Here's how the part is built. I have some questions about the finished solid (model axes, mm). A direction names the side the tool comes from. Round coordinates to 2 decimals unless told otherwise and drop trailing zeros. Loops run counter-clockwise (first coordinate to the right, second up) from the corner with the lowest first, then second, coordinate; pieces in that order, holes last. Notation, with made-up numbers: (2, 58.25) - (32, 58.25) arc R6 ccw to (32, 68.25) - close; hole circle Ø3 at (3.25, 74.25). An arc over 180 degrees is marked (long way). Return JSON: item names as keys, results as strings. Group by question number.
```python
from build123d import *

# Parameters (mm, degrees)
SKETCH1_R           = 1.5
BOSS_EXTRUDE1_DEPTH = 10
SKETCH2_R           = 4
BOSS_EXTRUDE2_DEPTH = 3
SKETCH3_W           = 1.5
SKETCH3_H           = 1
SKETCH3_W_2         = 1
SKETCH3_H_2         = 1.5
CUT_EXTRUDE1_DEPTH  = 2
FILLET1_SIZE        = 2
FILLET1_SIZE_2      = 3.5


with BuildPart() as part:
    # Sketch1 → Boss-Extrude1 (new body)
    with BuildSketch(Plane(origin=(0, 0, 0), x_dir=(1, 0, 0), z_dir=(0, 1, 0))):
        with Locations(Location((0, 0, 0), (0, 0, 270))):
            Circle(SKETCH1_R)
    extrude(amount=BOSS_EXTRUDE1_DEPTH)

    # Sketch2 → Boss-Extrude2 (add)
    with BuildSketch(Plane(origin=(0, 10, 0), x_dir=(1, 0, 0), z_dir=(0, 1, 0))):
        with Locations(Location((0, 0, 0), (0, 0, 270))):
            Circle(SKETCH2_R)
    extrude(amount=BOSS_EXTRUDE2_DEPTH)

    # Sketch3 → Cut-Extrude1 (cut)
    with BuildSketch(Plane(origin=(0, 13, 0), x_dir=(1, 0, 0), z_dir=(0, 1, 0))):
        with Locations((-1.25, 0)):
            Rectangle(SKETCH3_W, SKETCH3_H)
        Rectangle(SKETCH3_W_2, SKETCH3_H)
        with Locations((0, 1.25)):
            Rectangle(SKETCH3_W_2, SKETCH3_H_2)
        with Locations((1.25, 0)):
            Rectangle(SKETCH3_W, SKETCH3_H)
        with Locations((0, -1.25)):
            Rectangle(SKETCH3_W_2, SKETCH3_H_2)
    extrude(amount=-CUT_EXTRUDE1_DEPTH, mode=Mode.SUBTRACT)

    # Fillet1
    # an asymmetric fillet: 3.5, 2 mm, written as the material it takes off along each edge
    with BuildSketch(Plane(origin=(0, 13, 0), x_dir=(0, 0, 1), z_dir=(-1, 0, 0))) as fillet1_piece_1:
        with BuildLine():
            Bezier((4, -FILLET1_SIZE), (4, 0), (4 - FILLET1_SIZE_2, 0), weights=[1, 0.707106781, 1])
            Line((4 - FILLET1_SIZE_2, 0), (4, 0))
            Line((4, 0), (4, -FILLET1_SIZE))
        make_face()
    revolve(axis=Axis((0, 13, 0), (0, 1, 0)), mode=Mode.SUBTRACT)


solid = part.part
```
Q1. For faces 4 (the flat face through (0, 12, 2)), 5 (the cylindrical face through (-3.905, 10.493, -0.867)), which set-ups out of +Z, -Z, +X, -X, +Y, -Y let a thin tool reach every point of the face, with its end or its side?
Q2. Please list where these lines run through material, in increasing order: line 1 (X direction, y = 11.5, z = 1.5); line 2 (Y direction, x = -1, z = 0); line 3 (X direction, y = 4, z = 0).
Q3. Imagine slicing it at A-A, the plane y = 7.5. List the corners of the cut face in (x, z) for me.
Q4. If we mould it in two halves opening along Z, with no side actions, what happens to faces 1 (the flat face through (2, 12, 0)), 2 (the cylindrical face through (0.45, 4.93, 1.43)), 3 (the flat face through (0, 10, 2))? For each: +Z half, -Z half, draft (parallel to the pull), parting line (faces both ways), or undercut.
Q5. Will these pins go through, and if not, where does the flat tip stop? pin 1 Ø1 at (y, z) = (3, -1) entering from +X; pin 2 Ø0.8 at (y, z) = (12, -1.5) entering from -X; pin 3 Ø1.2 at (x, z) = (0, -1) entering from +Y.
Output values:
{
 "1": {"face 4": "+Y", "face 5": "+Y, -Y"},
 "2": {"line 1": "x = -3.59 to -0.5, 0.5 to 3.59", "line 2": "y = 0 to 11", "line 3": "x = -1.5 to 1.5"},
 "3": {"outline": "circle Ø3 at (0, 0)"},
 "4": {"face 1": "undercut", "face 2": "parting line", "face 3": "draft"},
 "5": {"pin 1": "stops at x = 1.41", "pin 2": "stops at x = -3.58", "pin 3": "stops at y = 12.99"}
}
